Check sheet for the modelled part. Datum: model origin and axes. Units: mm. A direction names the side the tool comes from. Round coordinates to 2 decimals unless told otherwise and drop trailing zeros. Order: outer loops, then holes, each group sorted by start corner. A loop starts at its lowest first (then second) coordinate and runs counter-clockwise, first axis right, second up.
```python
from build123d import *

# Parameters (mm, degrees)
EXTRUDE_1_DEPTH     = 20
SKETCH_2_W          = 20
SKETCH_2_H          = 20
CUT_EXTRUDE_1_DEPTH = 10


with BuildPart() as part:
    # 草圖1 → 填料-伸長1 (new body)
    with BuildSketch(Plane.XY):
        Polygon((-20, 10), (-25, 10), (-25, -10), (25, -10), (25, 10), (20, 10), (20, 0), (10, 0), (10, 10), (-10, 10), (-10, 0), (-20, 0), align=None)
    extrude(amount=EXTRUDE_1_DEPTH)

    # 草圖2 → 除料-伸長1 (cut)
    with BuildSketch(Plane(origin=(0, 0, 0), x_dir=(-1, 0, 0), z_dir=(0, 0, -1))):
        Rectangle(SKETCH_2_W, SKETCH_2_H)
    extrude(amount=-CUT_EXTRUDE_1_DEPTH, mode=Mode.SUBTRACT)


solid = part.part
```
Item 1: Access from +Z, -Z, +X, -X, +Y, -Y to the whole of each face (thin tool, end or side, straight path). Record for faces 5 (the flat face through (10, -5, 5)), 6 (the flat face through (15, 0, 10)), 7 (the flat face through (25, 0, 10)).
Answer:
face 5: -Z, +Y, -Y
face 6: +Z, -Z, +Y
face 7: +Z, -Z, +X, +Y, -Y
Item 2: Go/stop test with flat-tipped pins: P1, Ø5, axis at x = 17, z = 6.5, coming from the +Y side; P2, Ø5, axis at x = 4, y = -2, coming from the -Z side. Record where each tip stops, or that it passes through.
Answer:
P1: stops at y = 0
P2: stops at z = 10
Item 3: Scan lines: line 1 along X through (y, z) = (1, 19.25); line 2 along X through (y, z) = (4.5, 4.5); line 3 along X through (y, z) = (-8.25, 3). Record each from-to range of solid material in increasing order.
Answer:
line 1: x = -25 to -20, -10 to 10, 20 to 25
line 2: x = -25 to -20, 20 to 25
line 3: x = -25 to -10, 10 to 25
Item 4: Release check for a two-part mould opening along X. For faces 1 (the flat face through (-15, 0, 10)), 2 (the flat face through (-20, 5, 10)), 3 (the flat face through (0, -2, 20)), 4 (the flat face through (-25, 0, 10)) record: released by +X, released by -X, zero draft, split by the parting line, or undercut.
Answer:
face 1: undercut
face 2: undercut
face 3: zero draft
face 4: released by -X
Item 5: Sectioned sample at D-D (y = -7.5). Record the cut outline in (x, z), and give its area (3 significant figures).
Answer:
outline: (-25, 0) - (-10, 0) - (-10, 10) - (10, 10) - (10, 0) - (25, 0) - (25, 20) - (-25, 20) - close
area: 800 mm2
Item 6: Sectioned sample at B-B (z = 3). Record the cut outline in (x, y).
Answer:
outline: (-25, -10) - (-10, -10) - (-10, 0) - (-20, 0) - (-20, 10) - (-25, 10) - close; (10, -10) - (25, -10) - (25, 10) - (20, 10) - (20, 0) - (10, 0) - close
Item 7: Sectioned sample at C-C (z = 14.5). Record the cut outline in (x, y), and give its area (3 significant figures).
Answer:
outline: (-25, -10) - (25, -10) - (25, 10) - (20, 10) - (20, 0) - (10, 0) - (10, 10) - (-10, 10) - (-10, 0) - (-20, 0) - (-20, 10) - (-25, 10) - close
area: 800 mm2
Item 8: Sectioned sample at A-A (y = 5.5). Record the cut outline in (x, z), and give its area (3 significant figures).
Answer:
outline: (-25, 0) - (-20, 0) - (-20, 20) - (-25, 20) - close; (-10, 10) - (10, 10) - (10, 20) - (-10, 20) - close; (20, 0) - (25, 0) - (25, 20) - (20, 20) - close
area: 400 mm2
